Can you work these out from the model? Positions are in its coordinate system, mm. A direction names the side the tool comes from. Give positions to 0.01 mm unless a question says otherwise; leave off trailing zeros. Write each loop counter-clockwise with the first axis right and the second up, starting at its lowest first coordinate (ties: lowest second). Pieces come first, ordered by that corner, then holes. Notation, with made-up numbers: (56, 40) -> (68, 40) arc R37 cw to (68, 76) -> close; hole circle Ø9 at (74, 13). An arc over 180 degrees is marked (long way). One line per item, written item: value.
from build123d import *

# Parameters (mm, degrees)
SM_BASE_FLANGE_1_DEPTH      = 35
SKETCH_7_W                  = 70.5268
SKETCH_7_H                  = 3
EXTRUDE_1_DEPTH             = 60
SKETCH_8_R                  = 3.1
CUT_EXTRUDE_1_DEPTH         = 128.804538261
SKETCH_9_R                  = 1.6
CUT_EXTRUDE_2_DEPTH         = 128.804538261
PATTERN_CIRCULAR_1_COUNT    = 4
SKETCH_10_W                 = 20.5
SKETCH_10_H                 = 40.5
CUT_EXTRUDE_3_DEPTH         = 110.498858442
SKETCH_11_R                 = 2.1
CUT_EXTRUDE_4_DEPTH         = 110.498858442
PATTERN_LINEAR_1_COUNT      = 2
PATTERN_LINEAR_1_PITCH      = 10
PATTERN_LINEAR_1_COUNT_DIR2 = 2
PATTERN_LINEAR_1_PITCH_DIR2 = 49.5
SKETCH_14_R                 = 5.55
CUT_EXTRUDE_7_DEPTH         = 109.494239478
FILLET_1_R                  = 1
CHAMFER_4_SIZE              = 3
CHAMFER_5_SIZE              = 6
SKETCH_15_R                 = 1.6
CUT_EXTRUDE_8_DEPTH         = 110.498858442
SKETCH_16_R                 = 1.6
CUT_EXTRUDE_9_DEPTH         = 110.498858442
PATTERN_LINEAR_2_COUNT      = 2
PATTERN_LINEAR_2_PITCH      = 60


# Sheet-metal steps are written as plain solids
with BuildPart() as part:
    # Sketch 2 → 基材-凸緣1 (new body)
    with BuildSketch(Plane.XY):
        with BuildLine():
            Line((36, 35), (36, 0.7366))
            ThreePointArc((36, 0.7366), (35.784254855, 0.215745145), (35.2634, 0))
            Line((35.2634, 0), (-35.2634, 0))
            ThreePointArc((-35.2634, 0), (-35.784254855, 0.215745145), (-36, 0.7366))
            Line((-36, 0.7366), (-36, 35))
            Line((-36, 35), (-39, 35))
            Line((-39, 35), (-39, 0.7366))
            ThreePointArc((-39, 0.7366), (-37.905575199, -1.905575199), (-35.2634, -3))
            Line((-35.2634, -3), (35.2634, -3))
            ThreePointArc((35.2634, -3), (37.905575199, -1.905575199), (39, 0.7366))
            Line((39, 0.7366), (39, 35))
            Line((39, 35), (36, 35))
        make_face()
    extrude(amount=SM_BASE_FLANGE_1_DEPTH)

    # 草圖7 → 填料-伸長1 (add)
    with BuildSketch(Plane.XY.offset(35)):
        with Locations((0, -1.5)):
            Rectangle(SKETCH_7_W, SKETCH_7_H)
    extrude(amount=EXTRUDE_1_DEPTH)

    # 草圖8 → 除料-伸長1 (cut, through all)
    with BuildSketch(Plane(origin=(39, 0, 0), x_dir=(0, 0, -1), z_dir=(1, 0, 0))):
        with Locations(Location((-17.5, 17.5, 0), (0, 0, 90))):
            Circle(SKETCH_8_R)
    extrude(amount=-CUT_EXTRUDE_1_DEPTH, mode=Mode.SUBTRACT)

    # 草圖9 → 除料-伸長2 (cut, through all)
    with BuildSketch(Plane.ZY.offset(39)):
        with Locations((17.5, 7.5)):
            Circle(SKETCH_9_R)
    cut_extrude_2 = extrude(amount=-CUT_EXTRUDE_2_DEPTH, mode=Mode.SUBTRACT)

    # 環狀複製排列1: 除料-伸長2 ×4 about axis
    pattern_circular_1_axis = Axis((0, 17.5, 17.5), (1, 0, 0))
    for i in range(1, PATTERN_CIRCULAR_1_COUNT):
        add(cut_extrude_2.rotate(pattern_circular_1_axis, i * 360 / PATTERN_CIRCULAR_1_COUNT), mode=Mode.SUBTRACT)

    # 草圖10 → 除料-伸長3 (cut, through all)
    with BuildSketch(Plane.XZ.offset(3)):
        with Locations((-16.9, 64.85)):
            Rectangle(SKETCH_10_W, SKETCH_10_H)
    extrude(amount=-CUT_EXTRUDE_3_DEPTH, mode=Mode.SUBTRACT)

    # 草圖11 → 除料-伸長4 (cut, through all)
    with BuildSketch(Plane.XZ.offset(3)):
        with Locations((-21.9, 89.6)):
            Circle(SKETCH_11_R)
    cut_extrude_4 = extrude(amount=-CUT_EXTRUDE_4_DEPTH, mode=Mode.SUBTRACT)

    # 直線複製排列1: Cut-Extrude 4 2 × 2
    with Locations(*[(i * PATTERN_LINEAR_1_PITCH, 0, -j * PATTERN_LINEAR_1_PITCH_DIR2) for i in range(PATTERN_LINEAR_1_COUNT) for j in range(PATTERN_LINEAR_1_COUNT_DIR2) if (i, j) != (0, 0)]):
        add(cut_extrude_4, mode=Mode.SUBTRACT)

    # 草圖14 → 除料-伸長7 (cut, through all)
    with BuildSketch(Plane(origin=(0, 0, 0), x_dir=(1, 0, 0), z_dir=(0, 1, 0))):
        with Locations(Location((17.0034, -75, 0), (0, 0, 180))):
            Circle(SKETCH_14_R)
    extrude(amount=-CUT_EXTRUDE_7_DEPTH, mode=Mode.SUBTRACT)

    # 圓角1
    fillet_1_edges = [part.edges().sort_by_distance(p)[0] for p in [
        (-6.65, -1.5, 85.1),
        (-6.65, -1.5, 44.6),
        (-27.15, -1.5, 44.6),
        (-27.15, -1.5, 85.1),
    ]]
    fillet(fillet_1_edges, radius=FILLET_1_R)

    # 導角4
    chamfer_4_edges = [part.edges().sort_by_distance(p)[0] for p in [
        (-37.5, 35, 0),
        (37.5, 35, 0),
        (-37.5, 35, 35),
        (37.5, 35, 35),
    ]]
    chamfer(chamfer_4_edges, length=CHAMFER_4_SIZE)

    # 導角5
    chamfer_5_edges = [part.edges().sort_by_distance(p)[0] for p in [
        (35.2634, -1.5, 95),
        (-35.2634, -1.5, 95),
    ]]
    chamfer(chamfer_5_edges, length=CHAMFER_5_SIZE)

    # 草圖15 → 除料-伸長8 (cut, through all)
    with BuildSketch(Plane.XZ.offset(3)):
        with Locations((0, 90)):
            Circle(SKETCH_15_R)
    extrude(amount=-CUT_EXTRUDE_8_DEPTH, mode=Mode.SUBTRACT)

    # 草圖16 → 除料-伸長9 (cut, through all)
    with BuildSketch(Plane.XZ.offset(3)):
        with Locations((30, 35)):
            Circle(SKETCH_16_R)
    cut_extrude_9 = extrude(amount=-CUT_EXTRUDE_9_DEPTH, mode=Mode.SUBTRACT)

    # 直線複製排列2: 除料-伸長9 ×2
    with Locations(*[(-i * PATTERN_LINEAR_2_PITCH, 0, 0) for i in range(1, PATTERN_LINEAR_2_COUNT)]):
        add(cut_extrude_9, mode=Mode.SUBTRACT)


solid = part.part
1) Will these pins go through, and if not, where does the flat tip stop? pin 1 (2.5 mm diameter, centred on y = -2, z = 59, fed in from -X); pin 2 (2.5 mm diameter, centred on y = -1, z = 63, fed in from +X).
Answer list:
pin 1: stops at x = -35.26
pin 2: stops at x = 35.26
2) If we section it at B-B (z = 68): Write out the boundary of the cut face in (x, y), and give its area (3 significant figures).
Answer list:
outline: (-35.26, -3) -> (-27.15, -3) -> (-27.15, 0) -> (-35.26, 0) -> close; (-6.65, -3) -> (35.26, -3) -> (35.26, 0) -> (-6.65, 0) -> close
area: 150 mm^2
3) I need wall thicknesses on L1, parallel to Z at x = -21.9, y = -1; L2, parallel to X at y = 21.5, z = 33.5; L3, parallel to Y at x = 16, z = 15. Which ranges of each line are inside material? Lowest first, please.
Answer list:
L1: z = 0 to 38, 42.2 to 44.6, 85.1 to 87.5, 91.7 to 95
L2: x = -39 to -36, 36 to 39
L3: y = -3 to 0
4) We'd pull the mould along Y, two halves only. Please class faces 1 (the face through (37.48, 26.42, 18.68)), 2 (the face through (-39, 22, 17)), 3 (the face through (0, -3, 47)), 4 (the face through (38, 34, 2)): released by +Y, released by -Y, zero draft, split by the parting line, or undercut.
Answer list:
face 1: undercut
face 2: zero draft
face 3: released by -Y
face 4: released by +Y
5) If we section it at D-D (x = -21.9): Write out the boundary of the cut face in (y, z).
Answer list:
outline: (-3, 0) -> (0, 0) -> (0, 38) -> (-3, 38) -> close; (-3, 42.2) -> (0, 42.2) -> (0, 44.6) -> (-3, 44.6) -> close; (-3, 85.1) -> (0, 85.1) -> (0, 87.5) -> (-3, 87.5) -> close; (-3, 91.7) -> (0, 91.7) -> (0, 95) -> (-3, 95) -> close
6) If we section it at A-A (y = 4): Write out the boundary of the cut face in (x, z), and give its area (3 significant figures).
Answer list:
outline: (-39, 0) -> (-36, 0) -> (-36, 35) -> (-39, 35) -> close; (36, 0) -> (39, 0) -> (39, 35) -> (36, 35) -> close
area: 210 mm^2
7) If we section it at C-C (y = 17.5): State how many separate pieces and enclosed holes the cut face has, and give its area (3 significant figures).
Answer list:
separate pieces: 8
enclosed holes: 0
area: 134 mm^2
8) For faces 5 (the face through (-38, 15, 35)), 6 (the face through (-36, 18, 13)), 7 (the face through (-17, -2, 44.6)), which set-ups out of +Z, -Z, +X, -X, +Y, -Y let a thin tool reach every point of the face, with its end or its side?
Answer list:
face 5: +Z, -X, +Y, -Y
face 6: +Z, -Z, +Y
face 7: +Y, -Y
